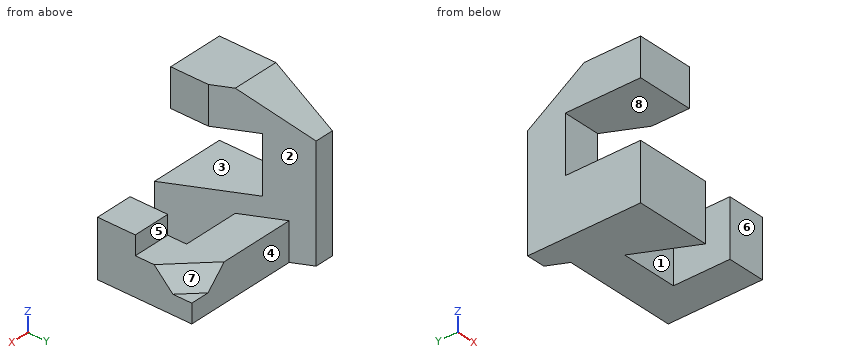
```python
from build123d import *

# Parameters (mm, degrees)
SKETCH1_W           = 4
SKETCH1_H           = 6
BOSS_EXTRUDE1_DEPTH = 8
SKETCH6_W           = 8
SKETCH6_H           = 6.708203932
CUT_EXTRUDE4_DEPTH  = 8
SKETCH7_W           = 3
SKETCH7_H           = 3
CUT_EXTRUDE5_DEPTH  = 10.433981132
SKETCH8_W           = 1
SKETCH8_H           = 2
CUT_EXTRUDE6_DEPTH  = 11.198039027
SKETCH9_W           = 3
SKETCH9_H           = 1
CUT_EXTRUDE7_DEPTH  = 10.433981132
CUT_EXTRUDE8_DEPTH  = 10.433981132
SKETCH12_W          = 2
SKETCH12_H          = 2
BOSS_EXTRUDE2_DEPTH = 3
SKETCH13_W          = 2
SKETCH13_H          = 2
BOSS_EXTRUDE3_DEPTH = 1.5
SKETCH14_W          = 2
SKETCH14_H          = 2
BOSS_EXTRUDE4_DEPTH = 3
SKETCH15_W          = 2
SKETCH15_H          = 2
BOSS_EXTRUDE5_DEPTH = 1
CUT_EXTRUDE9_DEPTH  = 1
CUT_EXTRUDE10_DEPTH = 1


with BuildPart() as part:
    # Sketch1 → Boss-Extrude1 (new body)
    with BuildSketch(Plane.XY):
        Rectangle(SKETCH1_W, SKETCH1_H)
    extrude(amount=BOSS_EXTRUDE1_DEPTH)

    # Sketch6 → Cut-Extrude4 (cut)
    with BuildSketch(Plane(origin=(0.4, 0.2, 0), x_dir=(0, 0, -1), z_dir=(0.894427190999916, 0.4472135954999579, 0))):
        with Locations((-4, -0.223606798)):
            Rectangle(SKETCH6_W, SKETCH6_H)
    extrude(amount=CUT_EXTRUDE4_DEPTH, mode=Mode.SUBTRACT)

    # Sketch7 → Cut-Extrude5 (cut, through all)
    with BuildSketch(Plane.ZY.offset(2)):
        with Locations((4.5, -1.5)):
            Rectangle(SKETCH7_W, SKETCH7_H)
    extrude(amount=-CUT_EXTRUDE5_DEPTH, mode=Mode.SUBTRACT)

    # Sketch8 → Cut-Extrude6 (cut, through all)
    with BuildSketch(Plane.XZ.offset(3)):
        with Locations((1.5, 7)):
            Rectangle(SKETCH8_W, SKETCH8_H)
    extrude(amount=-CUT_EXTRUDE6_DEPTH, mode=Mode.SUBTRACT)

    # Sketch9 → Cut-Extrude7 (cut, through all)
    with BuildSketch(Plane.ZY.offset(2)):
        with Locations((4.5, 0.5)):
            Rectangle(SKETCH9_W, SKETCH9_H)
    extrude(amount=-CUT_EXTRUDE7_DEPTH, mode=Mode.SUBTRACT)

    # Sketch10 → Cut-Extrude8 (cut, through all)
    with BuildSketch(Plane.ZY.offset(2)):
        Polygon((6, 3), (8, 0), (8, 3), align=None)
    extrude(amount=-CUT_EXTRUDE8_DEPTH, mode=Mode.SUBTRACT)

    # Sketch12 → Boss-Extrude2 (add, symmetric)
    with BuildSketch(Plane(origin=(1, 0, 0), x_dir=(0, 0, -1), z_dir=(1, 0, 0))):
        with Locations((-1, 1)):
            Rectangle(SKETCH12_W, SKETCH12_H)
    extrude(amount=BOSS_EXTRUDE2_DEPTH, both=True)

    # Sketch13 → Boss-Extrude3 (add)
    with BuildSketch(Plane(origin=(4, 0, 0), x_dir=(0, 0, -1), z_dir=(1, 0, 0))):
        with Locations((-1, 1)):
            Rectangle(SKETCH13_W, SKETCH13_H)
    extrude(amount=BOSS_EXTRUDE3_DEPTH)

    # Sketch14 → Boss-Extrude4 (add)
    with BuildSketch(Plane.XZ):
        with Locations((4.5, 1)):
            Rectangle(SKETCH14_W, SKETCH14_H)
    extrude(amount=BOSS_EXTRUDE4_DEPTH)

    # Sketch15 → Boss-Extrude5 (add)
    with BuildSketch(Plane.XY.offset(2)):
        with Locations((4.5, -2)):
            Rectangle(SKETCH15_W, SKETCH15_H)
    extrude(amount=BOSS_EXTRUDE5_DEPTH)

    # Sketch18 → Cut-Extrude9 (cut)
    with BuildSketch(Plane.XY.offset(2)):
        Polygon((5.5, 1), (4.5, 2), (5.5, 2), align=None)
    extrude(amount=-CUT_EXTRUDE9_DEPTH, mode=Mode.SUBTRACT)

    # 3DSketch1 → Cut-Extrude10 (cut, along a direction that is not the sketch's normal)
    with BuildSketch(Plane(origin=(5.5, 0, 2), x_dir=(-0.7071067811865472, 0.707106781186548, 0), z_dir=(-0.577350269189626, -0.5773502691896253, -0.5773502691896261))):
        Polygon((0, 0), (0.707106781, 1.224744871), (2.121320344, 1.224744871), (2.828427125, 0), align=None)
    extrude(amount=-CUT_EXTRUDE10_DEPTH, dir=(-0.7071067811865478, -0.7071067811865472, 0), mode=Mode.SUBTRACT)


solid = part.part
```
Input: part model. Units: mm. Frame: model coordinates. Face numbers are marked on the shaded views. A direction names the side the tool comes from. Give positions to 0.01 mm unless a question says otherwise; leave off trailing zeros. Order: outer loops, then holes, each group sorted by start corner. A loop starts at its lowest first (then second) coordinate and runs counter-clockwise, first axis right, second up. Notation, with made-up numbers: (-12.75, 35.25) -> (6.25, 35.25) arc R25 cw to (6.25, 69.25) -> close; hole circle Ø7 at (12.25, -13.5). An arc over 180 degrees is marked (long way). Write each question's results on one line, items separated by ' | '. Start each with the question number.
Item 1: Line query: line 1 (Y direction, x = 1.5, z = 1); line 2 (Z direction, x = 2.75, y = 0.75); line 3 (Y direction, x = 0.75, z = 6.75). Output: solid intervals per line, ascending.
Item 2: Mould query, pull axis Z, two halves, no side actions, for the marked faces 6, 7 and 8. Classes: pulls with the +Z half, pulls with the -Z half, needs draft (parallel to the pull), parting line crosses it, or undercut.
Item 3: Set-up query: the marked faces 1, 2, 3, 4 and 5. Return all of +Z, -Z, +X, -X, +Y, -Y with unobstructed straight access to the full face (end or side cutting, diameter ignored); none if empty.
Item 4: Cut plane B-B on x = 1.5. Return the cut outline in (y, z), then the cut area to 3 significant figures.
Item 5: Cut plane A-A on y = -2.5. Return the cut outline in (x, z).
Item 6: Contact query for flat-ended pins moving along their axis: P1, Ø1.5, axis at x = 4.5, y = 2, coming from the -Z side; P2, Ø1.6, axis at y = -2, z = 6.5, coming from the +X side; P3, Ø0.9, axis at x = 3.5, y = 0, coming from the +Z side; P4, Ø0.5, axis at x = 5, y = 1.5, coming from the +Z side. Output: stop coordinate, or through.
Item 7: Cut plane C-C on z = 1.5. Return the cut outline in (x, y).
Item 8: Cut plane D-D on y = 0.5. Return the cut outline in (x, z).
Established:
1) line 1: -3 to -2, 0 to 2 | line 2: 0 to 2 | line 3: -3 to -0.5
2) face 6: needs draft | face 7: pulls with the +Z half | face 8: undercut
3) face 1: +Z, -Z | face 2: +Z | face 3: +X, -X, -Y | face 4: +Z, -Z, +X, +Y | face 5: +Z, +X, +Y
4) outline: (-3, 0) -> (-2, 0) -> (-2, 3) -> (-3, 3) -> close; (0, 0) -> (2, 0) -> (2, 2) -> (0, 2) -> close | area: 7.00 mm^2
5) outline: (-2, 0) -> (1.75, 0) -> (1.75, 3) -> (-2, 3) -> close; (-2, 6) -> (1, 6) -> (1, 8) -> (-2, 8) -> close; (3.5, 0) -> (5.5, 0) -> (5.5, 3) -> (3.5, 3) -> close
6) P1: z = 0 | P2: x = 1 | P3: z = 2 | P4: z = 1.35
7) outline: (-2, -3) -> (2, -3) -> (0.5, 0) -> (3.5, 0) -> (3.5, -3) -> (5.5, -3) -> (5.5, 0.5) -> (4, 2) -> (-0.5, 2) -> (-1, 3) -> (-2, 3) -> close
8) outline: (-2, 0) -> (5.5, 0) -> (5.5, 1.5) -> (5, 2) -> (0.25, 2) -> (0.25, 3) -> (-2, 3) -> close; (-2, 6) -> (0.25, 6) -> (0.25, 7.67) -> (-2, 7.67) -> close
